Input: part model. Units: mm. Frame: model coordinates. Round coordinates to 2 decimals unless told otherwise and drop trailing zeros. Order: outer loops, then holes, each group sorted by start corner. A loop starts at its lowest first (then second) coordinate and runs counter-clockwise, first axis right, second up. Notation, with made-up numbers: M -4.75,-19.5 L 19.25,-19.5 A18 ccw 19.25,-11.5 Z; hole C 82,3 d11. An arc over 180 degrees is marked long. One line per question, with ' | ' between items.
```python
from build123d import *

# Parameters (mm, degrees)
MODEL_R         = 1
MODEL_R_2       = 1.5
EXTRUDE_1_DEPTH = 2


with BuildPart() as part:
    # Model → 凸台-拉伸1 (new body)
    with BuildSketch(Plane.XY):
        with BuildLine():
            ThreePointArc((165.794247794, 119.146851779), (178.48431443, 110.518191971), (193.458034411, 107.159729335))
            ThreePointArc((193.458034411, 107.159729335), (199.244879812, 100.139821501), (193.458034411, 93.119913668))
            ThreePointArc((193.458034411, 93.119913668), (178.48431443, 89.761451032), (165.794247794, 81.132791223))
            ThreePointArc((165.794247794, 81.132791223), (157.165587985, 68.442724587), (153.807125349, 53.469004606))
            ThreePointArc((153.807125349, 53.469004606), (146.787217515, 47.682159205), (139.767309682, 53.469004606))
            ThreePointArc((139.767309682, 53.469004606), (136.408847046, 68.442724587), (127.780187237, 81.132791223))
            ThreePointArc((127.780187237, 81.132791223), (115.090120601, 89.761451032), (100.11640062, 93.119913668))
            ThreePointArc((100.11640062, 93.119913668), (94.329555219, 100.139821501), (100.11640062, 107.159729335))
            ThreePointArc((100.11640062, 107.159729335), (115.090120601, 110.518191971), (127.780187237, 119.146851779))
            ThreePointArc((127.780187237, 119.146851779), (136.408847046, 131.836918416), (139.767309682, 146.810638396))
            ThreePointArc((139.767309682, 146.810638396), (146.787217515, 152.597483797), (153.807125349, 146.810638396))
            ThreePointArc((153.807125349, 146.810638396), (157.165587985, 131.836918416), (165.794247794, 119.146851779))
        make_face()
        with Locations((156.787217515, 110.139821501)):
            Circle(MODEL_R, mode=Mode.SUBTRACT)
        with Locations((136.787217515, 110.139821501)):
            Circle(MODEL_R, mode=Mode.SUBTRACT)
        with Locations((136.787217515, 90.139821501)):
            Circle(MODEL_R, mode=Mode.SUBTRACT)
        with Locations((156.787217515, 90.139821501)):
            Circle(MODEL_R, mode=Mode.SUBTRACT)
        with Locations((168.353974342, 100.139821501)):
            Circle(MODEL_R_2, mode=Mode.SUBTRACT)
        with Locations((146.787217515, 121.706578327)):
            Circle(MODEL_R_2, mode=Mode.SUBTRACT)
        with Locations((125.220460689, 100.139821501)):
            Circle(MODEL_R_2, mode=Mode.SUBTRACT)
        with Locations((146.787217515, 78.573064675)):
            Circle(MODEL_R_2, mode=Mode.SUBTRACT)
        with Locations((146.787217515, 126.706578327)):
            Circle(MODEL_R_2, mode=Mode.SUBTRACT)
        with Locations((120.220460689, 100.139821501)):
            Circle(MODEL_R_2, mode=Mode.SUBTRACT)
        with Locations((146.787217515, 73.573064675)):
            Circle(MODEL_R_2, mode=Mode.SUBTRACT)
        with Locations((173.353974342, 100.139821501)):
            Circle(MODEL_R_2, mode=Mode.SUBTRACT)
        with Locations((146.787217515, 118.171044401)):
            Circle(MODEL_R, mode=Mode.SUBTRACT)
        with Locations((128.755994615, 100.139821501)):
            Circle(MODEL_R, mode=Mode.SUBTRACT)
        with Locations((146.787217515, 82.108598601)):
            Circle(MODEL_R, mode=Mode.SUBTRACT)
        with Locations((164.818440415, 100.139821501)):
            Circle(MODEL_R, mode=Mode.SUBTRACT)
        with Locations((162.037217515, 115.389821501)):
            Circle(MODEL_R_2, mode=Mode.SUBTRACT)
        with Locations((131.537217515, 115.389821501)):
            Circle(MODEL_R_2, mode=Mode.SUBTRACT)
        with Locations((131.537217515, 84.889821501)):
            Circle(MODEL_R_2, mode=Mode.SUBTRACT)
        with Locations((162.037217515, 84.889821501)):
            Circle(MODEL_R_2, mode=Mode.SUBTRACT)
        with Locations((182.657217515, 100.139821501)):
            Circle(MODEL_R, mode=Mode.SUBTRACT)
        with Locations((146.787217515, 136.036864466)):
            Circle(MODEL_R, mode=Mode.SUBTRACT)
        with Locations((110.917217515, 100.139821501)):
            Circle(MODEL_R, mode=Mode.SUBTRACT)
        with Locations((146.787217515, 64.242778536)):
            Circle(MODEL_R, mode=Mode.SUBTRACT)
        with BuildLine():
            Line((152.398515146, 91.006916148), (141.004728844, 91.006916149))
            ThreePointArc((141.004728844, 91.006916149), (140.104214379, 91.379921453), (139.731209075, 92.280435918))
            ThreePointArc((139.731209075, 92.280435918), (140.104214379, 93.180950383), (141.004728844, 93.553955688))
            Line((141.004728844, 93.553955688), (152.398515146, 93.553955687))
            ThreePointArc((152.398515146, 93.553955687), (153.672034916, 92.280435917), (152.398515146, 91.006916148))
        make_face(mode=Mode.SUBTRACT)
        with BuildLine():
            Line((152.599718137, 109.199272945), (141.205931835, 109.199272945))
            ThreePointArc((141.205931835, 109.199272945), (140.30541737, 108.826267641), (139.932412066, 107.925753176))
            ThreePointArc((139.932412066, 107.925753176), (140.30541737, 107.025238711), (141.205931835, 106.652233406))
            Line((141.205931835, 106.652233406), (152.599718137, 106.652233406))
            ThreePointArc((152.599718137, 106.652233406), (153.873237907, 107.925753176), (152.599718137, 109.199272945))
        make_face(mode=Mode.SUBTRACT)
        with BuildLine():
            Line((151.898560909, 100.493374892), (147.140770906, 105.251164895))
            ThreePointArc((147.140770906, 105.251164895), (146.787217515, 105.397611504), (146.433664125, 105.251164895))
            Line((146.433664125, 105.251164895), (141.675874122, 100.493374892))
            ThreePointArc((141.675874122, 100.493374892), (141.529427512, 100.139821501), (141.675874122, 99.786268111))
            Line((141.675874122, 99.786268111), (146.433664125, 95.028478108))
            ThreePointArc((146.433664125, 95.028478108), (146.787217515, 94.882031498), (147.140770906, 95.028478108))
            Line((147.140770906, 95.028478108), (151.898560909, 99.786268111))
            ThreePointArc((151.898560909, 99.786268111), (152.045007518, 100.139821501), (151.898560909, 100.493374892))
        make_face(mode=Mode.SUBTRACT)
        with BuildLine():
            Line((137.779884988, 87.503468035), (155.779884988, 87.503468035))
            ThreePointArc((155.779884988, 87.503468035), (156.779884988, 86.503468035), (155.779884988, 85.503468035))
            Line((155.779884988, 85.503468035), (137.779884988, 85.503468035))
            ThreePointArc((137.779884988, 85.503468035), (137.072778206, 85.796361253), (136.779884988, 86.503468035))
            ThreePointArc((136.779884988, 86.503468035), (137.072778206, 87.210574816), (137.779884988, 87.503468035))
        make_face(mode=Mode.SUBTRACT)
        with BuildLine():
            Line((137.779884988, 112.776174968), (155.779884988, 112.776174968))
            ThreePointArc((155.779884988, 112.776174968), (156.779884988, 113.776174968), (155.779884988, 114.776174968))
            Line((155.779884988, 114.776174968), (137.779884988, 114.776174968))
            ThreePointArc((137.779884988, 114.776174968), (137.072778206, 114.483281749), (136.779884988, 113.776174968))
            ThreePointArc((136.779884988, 113.776174968), (137.072778206, 113.069068187), (137.779884988, 112.776174968))
        make_face(mode=Mode.SUBTRACT)
    extrude(amount=EXTRUDE_1_DEPTH)


solid = part.part
```
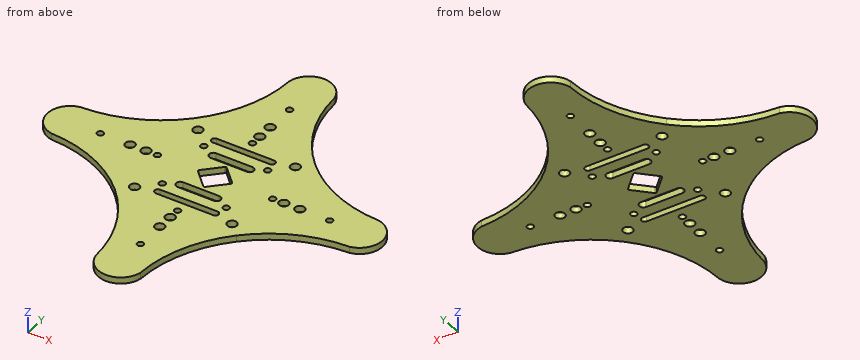
Item 1: Section query C-C, the plane y = 139.5. Return loops of the section in (x, z).
Report:
outline: M 138.87,0 L 154.71,0 L 154.71,2 L 138.87,2 Z
Item 2: First-contact query: pin 1 (1 mm diameter, centred on x = 151, z = 0.5, fed in from +Y); pin 2 (1 mm diameter, centred on x = 145.5, z = 1.5, fed in from +Y). Flat tips, straight axial feed; report the tip coordinate or a pass-through.
Report:
pin 1: y = 151.56 | pin 2: y = 152.55
Item 3: Section query B-B, the plane x = 185.5. Return loops of the section in (y, z).
Report:
outline: M 92.08,0 L 108.2,0 L 108.2,2 L 92.08,2 Z
Item 4: Section query A-A, the plane z = 1.7. Give the number of separate pieces and of enclosed holes in the cut face, plus the area to 3 significant figures.
Report:
separate pieces: 1 | enclosed holes: 29 | area: 3,780 mm²
Item 5: Line query: line 1 along Y through (x, z) = (150, 1.65); line 2 along Y through (x, z) = (163, 1.8); line 3 along X through (y, z) = (121.5, 1.6). Output: solid intervals per line, ascending. Write a range as from..to.
Report:
line 1: 48.44..85.5, 87.5..91.01, 93.55..97.89, 102.39..106.65, 109.2..112.78, 114.78..151.84 | line 2: 78.04..83.74, 86.04..114.24, 116.54..122.24 | line 3: 129.96..145.3, 148.27..163.62
